from build123d import *

# Parameters (mm, degrees)
SKETCH1_W            = 24
SKETCH1_H            = 44.45
BOSS_EXTRUDE1_DEPTH  = 20
M5_CLEARANCE_HOLE1_D = 5.5
BOSS_EXTRUDE2_START  = -20
SKETCH4_R            = 2.75
BOSS_EXTRUDE2_DEPTH  = 20
FILLET1_R            = 1
CHAMFER1_SIZE        = 0.25


with BuildPart() as part:
    # Sketch1 → Boss-Extrude1 (new body)
    with BuildSketch(Plane(origin=(0, 0, 0), x_dir=(1, 0, 0), z_dir=(0, 1, 0))):
        Rectangle(SKETCH1_W, SKETCH1_H)
    extrude(amount=BOSS_EXTRUDE1_DEPTH)

    # M5 Clearance Hole1 (through all)
    with Locations(Plane(origin=(0, 20, 0), x_dir=(1, 0, 0), z_dir=(0, 1, 0))):
        with Locations((-4.5, 15), (-4.5, -15), (-4.5, 0)):
            Hole(M5_CLEARANCE_HOLE1_D / 2)

    # Sketch4 → Boss-Extrude2 (add)
    with BuildSketch(Plane(origin=(0, 20, 0), x_dir=(1, 0, 0), z_dir=(0, 1, 0)).offset(BOSS_EXTRUDE2_START)):
        with Locations((-4.5, 0)):
            Circle(SKETCH4_R)
    extrude(amount=BOSS_EXTRUDE2_DEPTH)

    # Fillet1
    fillet1_edges = [part.edges().sort_by_distance(p)[0] for p in [
        (-12, 10, -22.225),
        (12, 10, -22.225),
        (12, 10, 22.225),
        (-12, 10, 22.225),
    ]]
    fillet(fillet1_edges, radius=FILLET1_R)

    # Chamfer1
    chamfer1_edges = [part.edges().sort_by_distance(p)[0] for p in [
        (-1.75, 20, 15),
        (-1.75, 0, 15),
        (-1.75, 20, -15),
        (-1.75, 0, -15),
        (-12, 0, 0),
        (-12, 20, 0),
        (0, 0, -22.225),
        (12, 0, 0),
        (0, 0, 22.225),
        (-11.707106781, 0, 21.932106781),
        (11.707106781, 0, 21.932106781),
        (11.707106781, 0, -21.932106781),
        (-11.707106781, 0, -21.932106781),
        (0, 20, -22.225),
        (0, 20, 22.225),
        (12, 20, 0),
        (-11.707106781, 20, 21.932106781),
        (11.707106781, 20, 21.932106781),
        (11.707106781, 20, -21.932106781),
        (-11.707106781, 20, -21.932106781),
    ]]
    chamfer(chamfer1_edges, length=CHAMFER1_SIZE)


solid = part.part
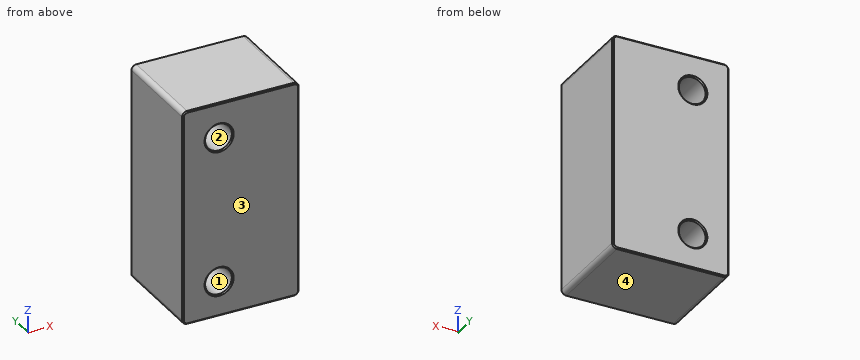
Geometry: final body of the model. Coordinates: model frame, mm. Face numbers are marked on the shaded views. Give positions to 0.01 mm unless a question says otherwise; leave off trailing zeros. Loops run counter-clockwise (first coordinate to the right, second up) from the corner with the lowest first, then second, coordinate; pieces in that order, holes last. Notation, with made-up numbers: (74, 40.5) - (118, 40.5) arc R25 cw to (118, 78.5) - close; hole circle Ø3 at (68, -1). An arc over 180 degrees is marked (long way). One line per question, with ' | ' between items. Start each with the question number.
(1) Pull-direction query (Z, two-part tool) for the marked faces 1, 2, 3 and 4; classes: released by +Z, released by -Z, zero draft, split by the parting line, or undercut.
(2) Section query C-C on x = -4.5. Return loops of the section in (y, z) (3 decimals).
(3) Section query B-B on y = 13. Return loops of the section in (x, z) (3 decimals).
(4) Section query A-A on z = 15. Return loops of the section in (x, y), then the cut area to 3 significant figures.
(5) Ray query, line 1 (Z direction, x = -4.5, y = 14.25) (3 decimals); line 2 (X direction, y = 11, z = 15); line 3 (X direction, y = 1, z = -12.5). Return the intervals inside material, ascending. Write a range as from..to.
(6) Contact query for a flat-ended pin moving along its axis: pin 1 (3.5 mm diameter, centred on x = -4.5, z = -15, fed in from +Y). Output: stop coordinate, or through.
The answers:
1) face 1: undercut | face 2: undercut | face 3: zero draft | face 4: released by -Z
2) outline: (0, -21.975) - (0.25, -22.225) - (19.75, -22.225) - (20, -21.975) - (20, -18) - (19.75, -17.75) - (0.25, -17.75) - (0, -18) - close; (0, -12) - (0.25, -12.25) - (19.75, -12.25) - (20, -12) - (20, 12) - (19.75, 12.25) - (0.25, 12.25) - (0, 12) - close; (0, 18) - (0.25, 17.75) - (19.75, 17.75) - (20, 18) - (20, 21.975) - (19.75, 22.225) - (0.25, 22.225) - (0, 21.975) - close
3) outline: (-12, -21.225) arc R1 ccw to (-11, -22.225) - (11, -22.225) arc R1 ccw to (12, -21.225) - (12, 21.225) arc R1 ccw to (11, 22.225) - (-11, 22.225) arc R1 ccw to (-12, 21.225) - close; hole circle Ø5.5 at (-4.5, -15); hole circle Ø5.5 at (-4.5, 15)
4) outline: (-12, 0.25) - (-11.75, 0) - (-7.5, 0) - (-7.25, 0.25) - (-7.25, 19.75) - (-7.5, 20) - (-11.75, 20) - (-12, 19.75) - close; (-1.75, 0.25) - (-1.5, 0) - (11.75, 0) - (12, 0.25) - (12, 19.75) - (11.75, 20) - (-1.5, 20) - (-1.75, 19.75) - close | area: 370 mm2
5) line 1: -22.225..-17.75, -12.25..12.25, 17.75..22.225 | line 2: -12..-7.25, -1.75..12 | line 3: -12..-5.65, -3.35..12
6) pin 1: through
